```python
from build123d import *

# Parameters (mm, degrees)
SKETCH4_W           = 30
SKETCH4_H           = 6
SKETCH4_W_2         = 6
SKETCH4_H_2         = 22
BOSS_EXTRUDE1_DEPTH = 140
SKETCH6_R           = 20
BOSS_EXTRUDE2_DEPTH = 10
SKETCH7_R           = 40
BOSS_EXTRUDE3_DEPTH = 10


with BuildPart() as part:
    # Sketch4 → Boss-Extrude1 (new body)
    with BuildSketch(Plane(origin=(1.761790339, -4.428283824, 0), x_dir=(1, 0, 0), z_dir=(0, 0, 1))):
        with Locations((-10.641284089, 16.5928688)):
            Rectangle(SKETCH4_W, SKETCH4_H)
        with Locations((-10.641284089, 2.5928688)):
            Rectangle(SKETCH4_W_2, SKETCH4_H_2)
        with Locations((-10.641284089, -11.4071312)):
            Rectangle(SKETCH4_W, SKETCH4_H)
    extrude(amount=BOSS_EXTRUDE1_DEPTH)

    # Sketch6 → Boss-Extrude2 (add)
    with BuildSketch(Plane(origin=(0, 0, 0), x_dir=(-1, 0, 0), z_dir=(0, 0, -1))):
        with Locations(Location((8.59379802, 0, 0), (0, 0, 137.367685303))):
            Circle(SKETCH6_R)
    extrude(amount=BOSS_EXTRUDE2_DEPTH)

    # Sketch7 → Boss-Extrude3 (add)
    with BuildSketch(Plane.XY.offset(140)):
        with Locations((-9.032018986, -1.718473877)):
            Circle(SKETCH7_R)
    extrude(amount=BOSS_EXTRUDE3_DEPTH)


solid = part.part
```
Design review of the part built by this model. Coordinates are the model's own, in mm. A direction names the side the tool comes from. Give positions to 0.01 mm unless a question says otherwise; leave off trailing zeros. Write each loop counter-clockwise with the first axis right and the second up, starting at its lowest first coordinate (ties: lowest second). Pieces come first, ordered by that corner, then holes.
(1) Tool access review of faces 1 (the face through (-22, -17, 0)), 2 (the face through (-23.879, 12, 69)), 3 (the face through (-1, -1, 140)): name each direction out of +Z, -Z, +X, -X, +Y, -Y from which nothing blocks a thin tool from reaching the whole face with its end or side.
Checked values:
face 1: -Z, -X, -Y
face 2: -X, +Y, -Y
face 3: none
(2) Clearance check with flat-ended pins moving along their axes: pin 1 Ø10 at (x, z) = (-8.5, 12) entering from -Y; pin 2 Ø17.5 at (y, z) = (-7.5, 43.5) entering from +X; pin 3 Ø6 at (y, z) = (-2.5, 89) entering from -X. State where each tip first meets the part, or that it passes through.
Checked values:
pin 1: stops at y = -18.84
pin 2: stops at x = 6.12
pin 3: stops at x = -11.88
(3) Add section A-A (x = 2). Give the boundary of the cut face in (y, z), and give its area (3 significant figures).
Checked values:
outline: (-40.17, 140) - (-18.84, 140) - (-18.84, 0) - (-16.96, 0) - (-16.96, -10) - (16.96, -10) - (16.96, 0) - (15.16, 0) - (15.16, 140) - (36.73, 140) - (36.73, 150) - (-40.17, 150) - close; hole (-12.84, 0) - (9.16, 0) - (9.16, 140) - (-12.84, 140) - close
area: 2,790 mm2
(4) Mouldability with a two-part tool opening along Z and no side actions: class faces 4 (the face through (4, -17, 0)), 5 (the face through (0, 9.165, 69)), 6 (the face through (-23.879, -16, 69)), 7 (the face through (-10, -1, 150)) as +Z half, -Z half, draft (parallel to the pull), parting line (faces both ways), or undercut.
Checked values:
face 4: -Z half
face 5: undercut
face 6: draft
face 7: +Z half
(5) Add section C-C (y = -16). Give the boundary of the cut face in (x, z), and give its area (3 significant figures).
Checked values:
outline: (-46.4, 140) - (-23.88, 140) - (-23.88, 0) - (-20.59, 0) - (-20.59, -10) - (3.41, -10) - (3.41, 0) - (6.12, 0) - (6.12, 140) - (28.33, 140) - (28.33, 150) - (-46.4, 150) - close
area: 5,190 mm2
(6) Add section B-B (z = 119.5). Give the boundary of the cut face in (x, y), and give its area (3 significant figures).
Checked values:
outline: (-23.88, -18.84) - (6.12, -18.84) - (6.12, -12.84) - (-5.88, -12.84) - (-5.88, 9.16) - (6.12, 9.16) - (6.12, 15.16) - (-23.88, 15.16) - (-23.88, 9.16) - (-11.88, 9.16) - (-11.88, -12.84) - (-23.88, -12.84) - close
area: 492 mm2
(7) Add section D-D (y = -26.5). Give the boundary of the cut face in (x, z).
Checked values:
outline: (-40.43, 140) - (22.37, 140) - (22.37, 150) - (-40.43, 150) - close
(8) Wall thickness on line 1 along Y through (x, z) = (-18.5, 45.5); line 2 along Z through (x, y) = (-27, -34); line 3 along X through (y, z) = (9, 58.5): over which ranges is each line inside the solid? List them lowest first.
Checked values:
line 1: y = -18.84 to -12.84, 9.16 to 15.16
line 2: z = 140 to 150
line 3: x = -11.88 to -5.88
